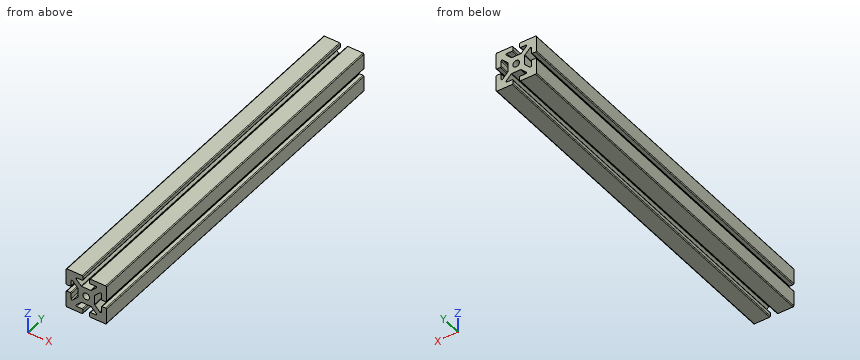
from build123d import *

# Parameters (mm, degrees)
SKETCH1_R           = 1
BOSS_EXTRUDE2_DEPTH = 55
FILLET2_R           = 0.25


with BuildPart() as part:
    # Sketch1 → Boss-Extrude2 (new body, symmetric)
    with BuildSketch(Plane(origin=(0, 0, 0), x_dir=(1, 0, 0), z_dir=(0, 1, 0))):
        Polygon((1, 6), (6, 6), (6, 1), (4.5, 1), (4.5, 3.439339828), (2.5, 1.439339828), (2.5, -1.439339828), (4.5, -3.439339828), (4.5, -1), (6, -1), (6, -6), (1, -6), (1, -4.5), (3.439339828, -4.5), (1.439339828, -2.5), (-1.439339828, -2.5), (-3.439339828, -4.5), (-1, -4.5), (-1, -6), (-6, -6), (-6, -1), (-4.5, -1), (-4.5, -3.439339828), (-2.5, -1.439339828), (-2.5, 1.439339828), (-4.5, 3.439339828), (-4.5, 1), (-6, 1), (-6, 6), (-1, 6), (-1, 4.5), (-3.439339828, 4.5), (-1.439339828, 2.5), (1.439339828, 2.5), (3.439339828, 4.5), (1, 4.5), align=None)
        Circle(SKETCH1_R, mode=Mode.SUBTRACT)
    extrude(amount=BOSS_EXTRUDE2_DEPTH, both=True)

    # Fillet2
    fillet2_edges = [part.edges().sort_by_distance(p)[0] for p in [
        (6, 0, -6),
        (6, 0, -1),
        (4.5, 0, -1),
        (4.5, 0, -3.439339828),
        (2.5, 0, -1.439339828),
        (2.5, 0, 1.439339828),
        (4.5, 0, 3.439339828),
        (4.5, 0, 1),
        (6, 0, 1),
        (6, 0, 6),
        (1, 0, 6),
        (1, 0, 4.5),
        (3.439339828, 0, 4.5),
        (1.439339828, 0, 2.5),
        (-1.439339828, 0, 2.5),
        (-3.439339828, 0, 4.5),
        (-1, 0, 4.5),
        (-1, 0, 6),
        (-6, 0, 6),
        (-6, 0, 1),
        (-4.5, 0, 1),
        (-4.5, 0, 3.439339828),
        (-2.5, 0, 1.439339828),
        (-2.5, 0, -1.439339828),
        (-4.5, 0, -3.439339828),
        (-4.5, 0, -1),
        (-6, 0, -1),
        (-6, 0, -6),
        (-1, 0, -6),
        (-1, 0, -4.5),
        (-3.439339828, 0, -4.5),
        (-1.439339828, 0, -2.5),
        (1.439339828, 0, -2.5),
        (3.439339828, 0, -4.5),
        (1, 0, -4.5),
        (1, 0, -6),
    ]]
    fillet(fillet2_edges, radius=FILLET2_R)


solid = part.part
Could you check a few things on this model? Use its own coordinates, in mm. Give positions to 0.01 mm unless a question says otherwise; leave off trailing zeros. Order: outer loops, then holes, each group sorted by start corner. A loop starts at its lowest first (then second) coordinate and runs counter-clockwise, first axis right, second up.
Item 1: I need wall thicknesses on line 1 (X direction, y = -14, z = -5.5); line 2 (Z direction, x = -1.5, y = -45); line 3 (X direction, y = 13, z = 0). Which ranges of each line are inside material? Lowest first, please.
Item 2: If we section it at B-B, the plane z = 0: Write out the boundary of the cut face in (x, y), plus the area to 3 significant figures.
Item 3: If we section it at A-A, the plane x = 0: Write out the boundary of the cut face in (y, z), plus the area to 3 significant figures.
Item 4: I'm going to push a flat-ended pin straight in: pin 1 (5 mm diameter, centred on y = -27.5, z = -1, fed in from +X). Where does the tip first touch, or does it pass through?
Values:
1. line 1: x = -6 to -1, 1 to 6
1. line 2: z = -6 to -4.5, -2.56 to 2.56, 4.5 to 6
1. line 3: x = -2.5 to -1, 1 to 2.5
2. outline: (-2.5, -55) - (-1, -55) - (-1, 55) - (-2.5, 55) - close; (1, -55) - (2.5, -55) - (2.5, 55) - (1, 55) - close
2. area: 330 mm2
3. outline: (-55, -2.5) - (55, -2.5) - (55, -1) - (-55, -1) - close; (-55, 1) - (55, 1) - (55, 2.5) - (-55, 2.5) - close
3. area: 330 mm2
4. pin 1: stops at x = 6
